Input: part model. Units: mm. Frame: model coordinates. A direction names the side the tool comes from. Round coordinates to 2 decimals unless told otherwise and drop trailing zeros. Loops run counter-clockwise (first coordinate to the right, second up) from the corner with the lowest first, then second, coordinate; pieces in that order, holes last.
(1) Cut plane A-A, the plane x = 17. Output: boundary loops of the cut face in (y, z), and give its area (3 significant figures).
(2) Line query: line 1 (Z direction, x = 5, y = 2.25); line 2 (X direction, y = 5.75, z = 70); line 3 (Z direction, x = 8.5, y = 6.25). Output: solid intervals per line, ascending.
(3) Cut plane C-C, the plane x = 3. Output: boundary loops of the cut face in (y, z).
(4) Cut plane B-B, the plane y = 2. Output: boundary loops of the cut face in (x, z) (3 decimals).
(5) Draft query along X for faces 4 (the face through (-18, 0, 60)), 5 (the face through (16.368, 3.131, 3.282)), 6 (the face through (7.573, 3.131, 9.091)). Return one class per face: released by +X, released by -X, zero draft, split by the parting line, or undercut.
(6) Access query for faces 1 (the face through (16.733, 3.131, 29.13)), 2 (the face through (0, 3, 13)), 3 (the face through (19.05, 3, 17)). Directions: +Z, -Z, +X, -X, +Y, -Y. A direction counts if a zero-diameter tool reaches every point of the face in a straight line with its end or side. Return the directions, or none.
(7) Cut plane D-D, the plane z = 59.5. Output: boundary loops of the cut face in (x, y).
(8) First-contact query: pin 1 Ø1.5 at (y, z) = (3, 108) entering from +X; pin 2 Ø1 at (x, y) = (-18.5, 3) entering from +Z; pin 3 Ø3 at (x, y) = (-9, 3) entering from +Z. Flat tips, straight axial feed; report the tip coordinate or a pass-through.
from build123d import *

# Parameters (mm, degrees)
SKETCH1_R           = 2
BOSS_EXTRUDE1_DEPTH = 6.35
FILLET1_R           = 10.16


with BuildPart() as part:
    # Sketch1 → Boss-Extrude1 (new body)
    with BuildSketch(Plane(origin=(0, 0, 0), x_dir=(1, 0, 0), z_dir=(0, 1, 0))):
        with BuildLine():
            Line((19.05, 0), (0, 0))
            Line((0, 0), (0, -22.757139607))
            ThreePointArc((0, -22.757139607), (-30.814603217, -79.553676933), (19.05, -120.65))
            ThreePointArc((19.05, -120.65), (25.4, -114.3), (19.05, -107.95))
            ThreePointArc((19.05, -107.95), (-19.05, -69.85), (19.05, -31.75))
            Line((19.05, -31.75), (19.05, 0))
        make_face()
        with Locations(Location((9.525, -9.525, 0), (0, 0, 270))):
            Circle(SKETCH1_R, mode=Mode.SUBTRACT)
        with Locations(Location((-12.380896424, -38.419103576, 0), (0, 0, 270))):
            Circle(SKETCH1_R, mode=Mode.SUBTRACT)
        with Locations(Location((-12.380896424, -101.280896424, 0), (0, 0, 270))):
            Circle(SKETCH1_R, mode=Mode.SUBTRACT)
    extrude(amount=BOSS_EXTRUDE1_DEPTH)

    # Fillet1
    # the kernel refuses this fillet: 10.16 mm, written as the material it adds along each edge
    with BuildSketch(Plane(origin=(0, 0, 22.757139607), x_dir=(0, 0, -1), z_dir=(0, 1, 0))) as fillet1_piece_1:
        with BuildLine():
            CenterArc((6.413190667, 10.16), FILLET1_R, 208.630989837, 61.369010163)
            ThreePointArc((-2.50448451, 5.291666667), (-1.175949507, 2.681941807), (0, 0))
            Line((0, 0), (6.413190667, 0))
        make_face()
    extrude(amount=6.35)
    # the kernel refuses this fillet: 10.16 mm, written as the material it takes off along each edge
    with BuildSketch(Plane(origin=(19.05, -22.696015193, 31.75), x_dir=(0, 0, -1), z_dir=(0, 1, 0))) as fillet1_2_piece_1:
        with BuildLine():
            CenterArc((9.078406077, 10.16), FILLET1_R, 192.153197469, 77.846802531)
            ThreePointArc((-0.853889939, 8.021052632), (-0.214073897, 4.033187739), (0, 0))
            Line((0, 0), (9.078406077, 0))
        make_face()
    extrude(amount=51.742030387, mode=Mode.SUBTRACT)
    with BuildSketch(Plane(origin=(0, -25.4, 0), x_dir=(1, 0, 0), z_dir=(0, 1, 0)), Plane(origin=(19.05, -25.4, 0), x_dir=(0, 0, 1), z_dir=(0, 1, 0))) as fillet1_2_piece_2:
        with BuildLine():
            CenterArc((FILLET1_R, -FILLET1_R), FILLET1_R, 90, 90)
            Line((0, -FILLET1_R), (0, 0))
            Line((0, 0), (FILLET1_R, 0))
        make_face()
    extrude(amount=57.15, mode=Mode.SUBTRACT)


solid = part.part
Reported:
1. outline: (0, 4.04) - (6.35, 4.04) - (6.35, 28.79) - (0, 28.79) - close; (0, 107.89) - (6.35, 107.89) - (6.35, 120.61) - (0, 120.61) - close
1. area: 238 mm2
2. line 1: z = 1.41 to 34.44, 105.26 to 118.67
2. line 2: x = -31.75 to -19.05
2. line 3: z = 0.14 to 7.81, 11.24 to 33.24, 106.46 to 119.54
3. outline: (0, 2.95) - (6.35, 2.95) - (6.35, 35.3) - (0, 35.3) - close; (0, 104.4) - (6.35, 104.4) - (6.35, 118.05) - (0, 118.05) - close
4. outline: (-5.292, 25.262) arc R10.16 cw to (0, 16.344) - (0, 10.16) arc R10.16 ccw to (9.525, 0.02) arc R10.16 ccw to (19.05, 10.16) - (19.05, 22.672) arc R10.16 ccw to (11.029, 32.604) arc R38.1 cw to (19.05, 107.95) arc R6.35 ccw to (19.05, 120.65) arc R50.8 ccw to start; hole circle Ø4 at (-12.381, 38.419); hole circle Ø4 at (-12.381, 101.281); hole circle Ø4 at (9.525, 9.525)
5. face 4: zero draft
5. face 5: released by +X
5. face 6: undercut
6. face 1: +X, +Y, -Y
6. face 2: -Z, -X, +Y, -Y
6. face 3: -Z, +X, +Y, -Y
7. outline: (-30.68, 0) - (-17.62, 0) - (-17.62, 6.35) - (-30.68, 6.35) - close
8. pin 1: stops at x = 22.14
8. pin 2: stops at z = 104.61
8. pin 3: stops at z = 113.16
